Could you check a few things on this model? Use its own coordinates, in mm. Face numbers are marked on the shaded views. A direction names the side the tool comes from. Give positions to 0.01 mm unless a question says otherwise; leave off trailing zeros. Order: outer loops, then holes, each group sorted by start corner. A loop starts at its lowest first (then second) coordinate and runs counter-clockwise, first axis right, second up. Notation, with made-up numbers: M 58.5,87.25 L 87.5,87.25 A11 ccw 87.5,100.25 Z; hole C -27,-6 d8. An arc over 180 degrees is marked long. Use a Markdown table: item, result. Add a question column.
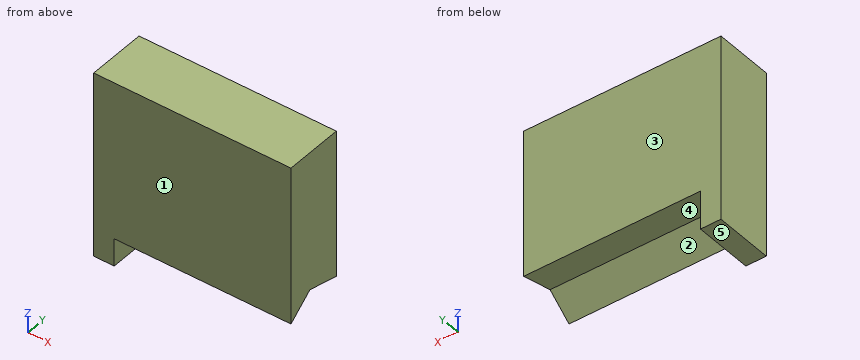
```python
from build123d import *

# Parameters (mm, degrees)
F0_W     = 134.338587
F0_H     = 40.145545
F1_DEPTH = 127
F3_DEPTH = 120.391601


with BuildPart() as f1:
    # F0 (on Top) → F1 (new body)
    with BuildSketch(Plane.XY):
        with Locations((53.221307, -3.590211)):
            Rectangle(F0_W, F0_H)
    extrude(amount=F1_DEPTH)

    # F2 (on Right) → F3 (cut, through all)
    with BuildSketch(Plane.YZ):
        Polygon((20.078405, -25.822868), (32.707811, -0.402366), (20.707569, 25.321126), (-6.885895, 31.977293), (-29.29414, 14.553907), (-29.6433, -13.828869), (-7.67045, -31.798224), align=None)
    extrude(amount=F3_DEPTH, mode=Mode.SUBTRACT)


solid = f1.part
```
1) Suppose I cut it at A-A on x = 108.5. Please give me the cut outline in (y, z), and give its area (3 significant figures).
2) For pin 1 (12 mm diameter, centred on x = 71.5, y = -4, fed in from -Z); pin 2 (12 mm diameter, centred on x = 98.5, y = -1.5, fed in from -Z); pin 3 (9.5 mm diameter, centred on y = -5, z = 12, fed in from +X), each with a flat end and sliding along its axis, tell me the tip position at first contact or that it passes through.
3) For the marked faces 1 and 2, which set-ups out of +Z, -Z, +X, -X, +Y, -Y let a thin tool reach every point of the face, with its end or its side?
4) We'd pull the mould along Y, two halves only. Please class the marked faces 3, 4 and 5: pulls with the +Y half, pulls with the -Y half, needs draft (parallel to the pull), parting line crosses it, or undercut.
5) Suppose I cut it at C-C on y = -17. Please give me the cut outline in (x, z).
6) Suppose I cut it at B-B on z = 12. Please give me the cut outline in (x, y), and give its area (3 significant figures).
7) Please list where these lines run through material, in increasing order: line 1 (X direction, y = -10.5, z = 16); line 2 (Z direction, x = 55.5, y = 3); line 3 (Z direction, x = 97, y = -19). Write a range as from..to.
8) Suppose I cut it at D-D on y = 11.5. Please give me the cut outline in (x, z).
Values found:
| question | item | result |
|---|---|---|
| 1 | outline | M -23.66,18.93 L -6.89,31.98 L 16.48,26.34 L 16.48,127 L -23.66,127 Z |
| 1 | area | 3,990 mm^2 |
| 2 | pin 1 | stops at z = 29.56 |
| 2 | pin 2 | stops at z = 29.23 |
| 2 | pin 3 | stops at x = 0 |
| 3 | face 1 | +Z, -Z, +X, -X, -Y |
| 3 | face 2 | -Z, +X |
| 4 | face 3 | pulls with the +Y half |
| 4 | face 4 | undercut |
| 4 | face 5 | needs draft |
| 5 | outline | M -13.95,0 L 0,0 L 0,24.11 L 120.39,24.11 L 120.39,127 L -13.95,127 Z |
| 6 | outline | M -13.95,-23.66 L 0,-23.66 L 0,16.48 L -13.95,16.48 Z |
| 6 | area | 560 mm^2 |
| 7 | line 1 | x = -13.95..0 |
| 7 | line 2 | z = 29.59..127 |
| 7 | line 3 | z = 22.56..127 |
| 8 | outline | M -13.95,0 L 0,0 L 0,27.54 L 120.39,27.54 L 120.39,127 L -13.95,127 Z |
